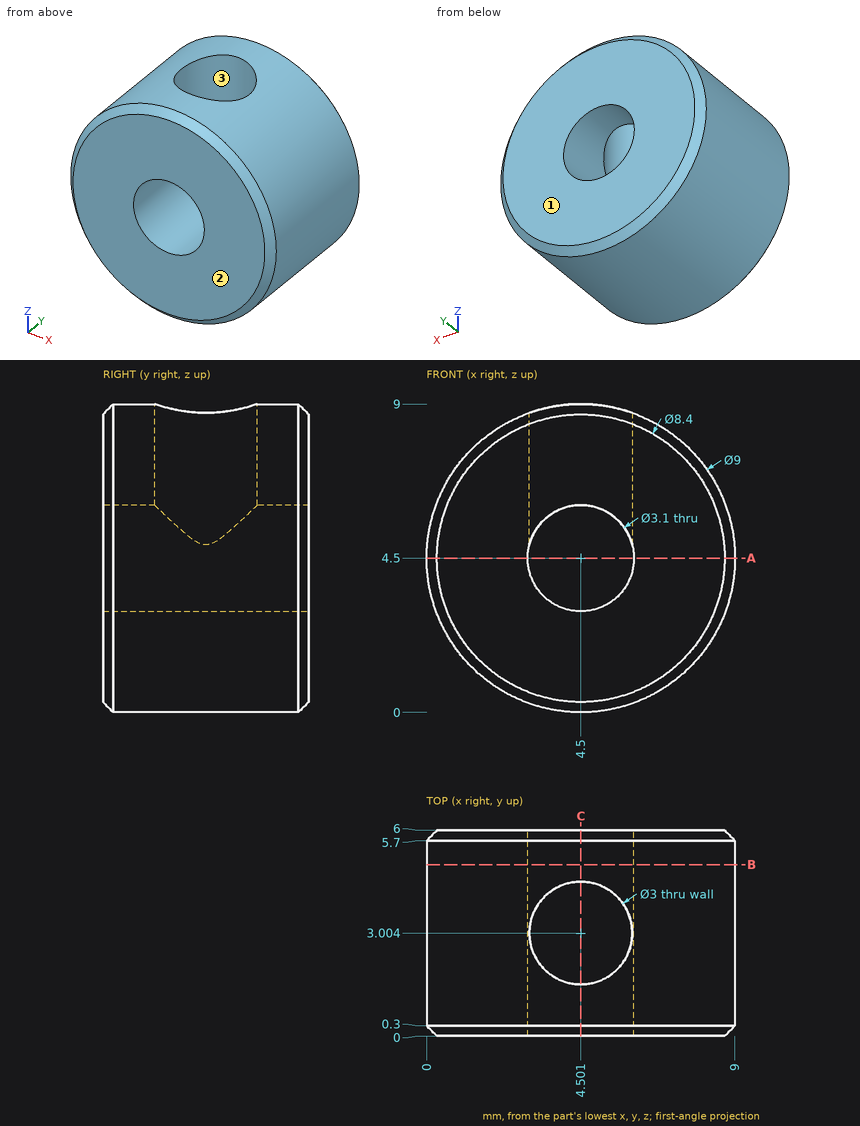
Answer from the drawing. Dimensions are ordinates in mm from the lowest x, y and z of the part. Coordinates: 2 decimals unless noted, no trailing zeros. Order: outer loops, then holes, each group sorted by start corner. A loop starts at its lowest first (then second) coordinate and runs counter-clockwise, first axis right, second up. Notation, with made-up numbers: (76.25, 13) - (81.25, 13) arc R9 ccw to (81.25, 24) - close; hole circle Ø3 at (69, 74.5). An arc over 180 degrees is marked (long way). Answer as a JSON object with one key per item and string values. Group by question number.
Item 1: Section A-A (z = 4.5) is taken. Give the vertices of the cut face in (x, y).
Item 2: A flat-ended cylindrical pin translates along its axis: P1, Ø5, axis at x = 4.5, z = 4.5, coming from the +Y side. Find the tip coordinate at first contact, or state that the pin passes through.
Item 3: Section C-C (x = 4.5) is taken. State how many separate pieces and enclosed holes the cut face has.
Item 4: Section B-B (y = 5) is taken. Give the vertices of the cut face in (x, z).
Item 5: The mould has two halves that part along Y. Classify the marked faces 1, 2 and 3: +Y half, -Y half, draft (parallel to the pull), parting line (faces both ways), or undercut.
Item 6: Consider probe 1 along X at (y, z) = (0.75, 4.5); probe 2 along Y at (x, z) = (5.25, 8) (1 decimal); probe 3 along Y at (x, z) = (5.75, 5.5) (1 decimal). Determine where each line is inside the solid, lowest interval first. Write a range as from..to.
Results are:
{
 "1": {"outline": "(0, 0.3) - (0.3, 0) - (2.95, 0) - (2.95, 6) - (0.3, 6) - (0, 5.7) - close; (6.05, 0) - (8.7, 0) - (9, 0.3) - (9, 5.7) - (8.7, 6) - (6.05, 6) - close"},
 "2": {"P1": "stops at y = 6"},
 "3": {"separate pieces": "3", "enclosed holes": "0"},
 "4": {"outline": "circle Ø9 at (4.5, 4.5); hole circle Ø3.1 at (4.5, 4.5)"},
 "5": {"face 1": "+Y half", "face 2": "-Y half", "face 3": "undercut"},
 "6": {"probe 1": "x = 0..2.95, 6.05..9", "probe 2": "y = 0..1.7, 4.3..6", "probe 3": "y = 0..2.2, 3.8..6"}
}
